from build123d import *

# Parameters (mm, degrees)
F0_R     = 1.5
F1_DEPTH = 2


with BuildPart() as f1:
    # F0 (on Top) → F1 (new body)
    with BuildSketch(Plane.XY):
        with BuildLine():
            ThreePointArc((27.5, 39.5), (26.62132, 41.62132), (24.5, 42.5))
            Line((24.5, 42.5), (-24.5, 42.5))
            ThreePointArc((-24.5, 42.5), (-26.62132, 41.62132), (-27.5, 39.5))
            Line((-27.5, 39.5), (-27.5, -39.5))
            ThreePointArc((-27.5, -39.5), (-26.62132, -41.62132), (-24.5, -42.5))
            Line((-24.5, -42.5), (24.5, -42.5))
            ThreePointArc((24.5, -42.5), (26.62132, -41.62132), (27.5, -39.5))
            Line((27.5, -39.5), (27.5, 39.5))
        make_face()
        with Locations((24.5, -39.5)):
            Circle(F0_R, mode=Mode.SUBTRACT)
        with BuildLine():
            Line((14, 19.5), (14, 13.833333))
            ThreePointArc((14, 13.833333), (13.645354, 12.418377), (12.665265, 11.337959))
            ThreePointArc((12.665265, 11.337959), (6.617002, 8.48056), (0, 7.5))
            ThreePointArc((0, 7.5), (-6.617002, 8.48056), (-12.665265, 11.337959))
            ThreePointArc((-12.665265, 11.337959), (-13.645354, 12.418377), (-14, 13.833333))
            Line((-14, 13.833333), (-14, 19.5))
            ThreePointArc((-14, 19.5), (-13.12132, 21.62132), (-11, 22.5))
            Line((-11, 22.5), (0, 22.5))
            Line((0, 22.5), (11, 22.5))
            ThreePointArc((11, 22.5), (13.12132, 21.62132), (14, 19.5))
        make_face(mode=Mode.SUBTRACT)
    extrude(amount=F1_DEPTH)


solid = f1.part
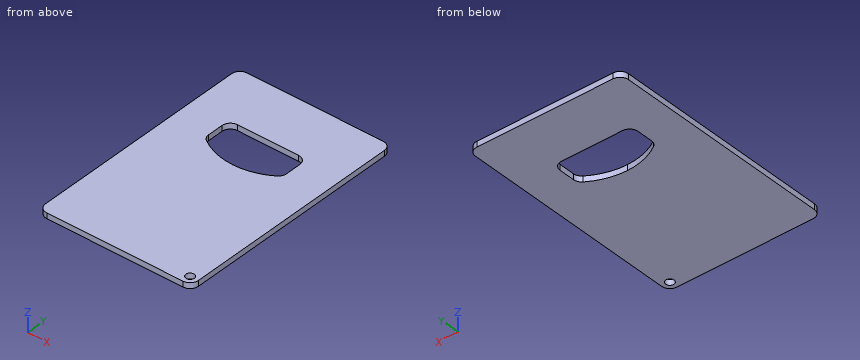
Check sheet for the modelled part. Datum: model origin and axes. Units: mm. Round coordinates to 2 decimals unless told otherwise and drop trailing zeros. Write each loop counter-clockwise with the first axis right and the second up, starting at its lowest first coordinate (ties: lowest second). Pieces come first, ordered by that corner, then holes. Notation, with made-up numbers: (45, 58.5) -> (79, 58.5) arc R19 cw to (79, 78.5) -> close; hole circle Ø3 at (68.25, 89). An arc over 180 degrees is marked (long way). Answer as CSV lines item,"result". Start each with the question number.
1) Material ranges on line 1 (X direction, y = 18, z = 1.1); line 2 (Y direction, x = 24.5, z = 0.5); line 3 (X direction, y = -38.5, z = 1.65), recorded low to high. Write a range as from..to.
2) Section check A-A on z = 1.1. Enter the section's corners in (x, y), and give its area (3 significant figures).
3) Section check B-B on y = 13. Enter the section's corners in (x, z).
Found:
1,line 1,"x = -27.5..-14, 14..27.5"
1,line 2,"y = -42.5..-41, -38..42.5"
1,line 3,"x = -27.5..23.38, 25.62..27.5"
2,outline,"(-27.5, -39.5) arc R3 ccw to (-24.5, -42.5) -> (24.5, -42.5) arc R3 ccw to (27.5, -39.5) -> (27.5, 39.5) arc R3 ccw to (24.5, 42.5) -> (-24.5, 42.5) arc R3 ccw to (-27.5, 39.5) -> close; hole (-14, 13.83) arc R3 ccw to (-12.67, 11.34) arc R22.82 ccw to (0, 7.5) arc R22.82 ccw to (12.67, 11.34) arc R3 ccw to (14, 13.83) -> (14, 19.5) arc R3 ccw to (11, 22.5) -> (-11, 22.5) arc R3 ccw to (-14, 19.5) -> close; hole circle Ø3 at (24.5, -39.5)"
2,area,"4,290 mm^2"
3,outline,"(-27.5, 0) -> (-13.88, 0) -> (-13.88, 2) -> (-27.5, 2) -> close; (13.88, 0) -> (27.5, 0) -> (27.5, 2) -> (13.88, 2) -> close"
